Geometry: final body of the model. Coordinates: model frame, mm. Give positions to 0.01 mm unless a question says otherwise; leave off trailing zeros. Write each loop counter-clockwise with the first axis right and the second up, starting at its lowest first coordinate (ties: lowest second). Pieces come first, ordered by that corner, then holes. Notation, with made-up numbers: (78.25, 77.5) -> (125.25, 77.5) arc R13 cw to (125.25, 91.5) -> close; hole circle Ø5 at (-17.5, -35). An arc over 180 degrees is marked (long way). Answer in a Markdown table with one row per item. Add a question column.
Item 1: Section query B-B on x = 12.5. Output: boundary loops of the cut face in (y, z).
Item 2: Material intervals for probe 1 along Y at (x, z) = (18.25, -19.05); probe 2 along Z at (x, y) = (15, 402); probe 3 along Y at (x, z) = (1.5, -12), sorted ascending. Write a range as from..to.
Item 3: Section query A-A on y = 438.15. Output: boundary loops of the cut face in (x, z), plus the area to 3 significant figures.
Item 4: Section query C-C on z = -19.05. Output: boundary loops of the cut face in (x, y).
Item 5: First-contact query: P1, Ø10, axis at x = 8, z = -19.5, coming from the -Y side. Flat tip, straight axial feed; report the tip coordinate or a pass-through.
```python
from build123d import *

# Parameters (mm, degrees)
SKETCH1_W           = 19.05
SKETCH1_H           = 38.1
SKETCH1_W_2         = 15.875
SKETCH1_H_2         = 34.925
EXTRUDE_THIN1_DEPTH = 457.2
SKETCH3_W           = 19.05
SKETCH3_H           = 38.1
SKETCH3_W_2         = 15.875
SKETCH3_H_2         = 34.925
EXTRUDE_THIN2_DEPTH = 75.184
SKETCH4_R           = 14.2875
CUT_EXTRUDE1_DEPTH  = 20.05


with BuildPart() as part:
    # Sketch1 → Extrude-Thin1 (new body)
    with BuildSketch(Plane(origin=(0, 0, 0), x_dir=(1, 0, 0), z_dir=(0, 1, 0))):
        with Locations((9.525, 19.05)):
            Rectangle(SKETCH1_W, SKETCH1_H)
        with Locations((9.525, 19.05)):
            Rectangle(SKETCH1_W_2, SKETCH1_H_2, mode=Mode.SUBTRACT)
    extrude(amount=EXTRUDE_THIN1_DEPTH)

    # Sketch3 → Extrude-Thin2 (add)
    with BuildSketch(Plane(origin=(0, 0, 0), x_dir=(-1, 0, 0), z_dir=(0, -1, 0))):
        with Locations((-9.525, 19.05)):
            Rectangle(SKETCH3_W, SKETCH3_H)
        with Locations((-9.525, 19.05)):
            Rectangle(SKETCH3_W_2, SKETCH3_H_2, mode=Mode.SUBTRACT)
    extrude(amount=EXTRUDE_THIN2_DEPTH)

    # Sketch4 → Cut-Extrude1 (cut, through all)
    with BuildSketch(Plane(origin=(19.05, 0, 0), x_dir=(0, 0, -1), z_dir=(1, 0, 0))):
        with Locations((19.2024, 438.15)):
            Circle(SKETCH4_R)
        with Locations((19.05, 8.636)):
            Circle(SKETCH4_R)
    extrude(amount=-CUT_EXTRUDE1_DEPTH, mode=Mode.SUBTRACT)


solid = part.part
```
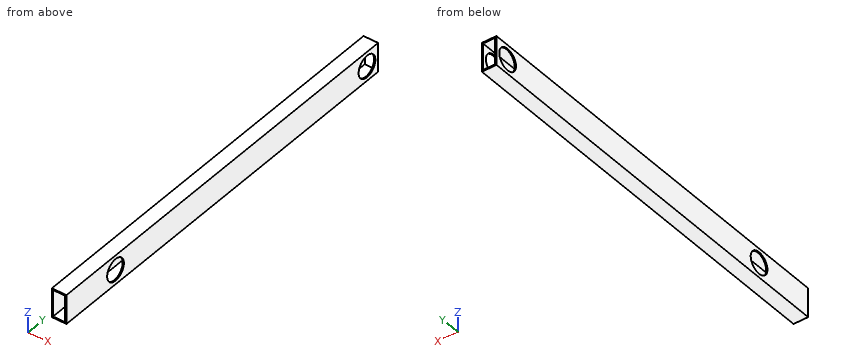
Findings below:
| question | item | result |
|---|---|---|
| 1 | outline | (-75.18, -38.1) -> (457.2, -38.1) -> (457.2, -36.51) -> (-75.18, -36.51) -> close; (-75.18, -1.59) -> (457.2, -1.59) -> (457.2, 0) -> (-75.18, 0) -> close |
| 2 | probe 1 | y = -75.18..-5.65, 22.92..423.86, 452.44..457.2 |
| 2 | probe 2 | z = -38.1..-36.51, -1.59..0 |
| 2 | probe 3 | y = -75.18..-3.79, 21.06..425.81, 450.49..457.2 |
| 3 | outline | (0, -38.1) -> (19.05, -38.1) -> (19.05, -33.49) -> (17.46, -33.49) -> (17.46, -36.51) -> (1.59, -36.51) -> (1.59, -33.49) -> (0, -33.49) -> close; (0, -4.91) -> (1.59, -4.91) -> (1.59, -1.59) -> (17.46, -1.59) -> (17.46, -4.91) -> (19.05, -4.91) -> (19.05, 0) -> (0, 0) -> close |
| 3 | area | 80.6 mm^2 |
| 4 | outline | (0, -75.18) -> (1.59, -75.18) -> (1.59, -5.65) -> (0, -5.65) -> close; (0, 22.92) -> (1.59, 22.92) -> (1.59, 423.86) -> (0, 423.86) -> close; (0, 452.44) -> (1.59, 452.44) -> (1.59, 457.2) -> (0, 457.2) -> close; (17.46, -75.18) -> (19.05, -75.18) -> (19.05, -5.65) -> (17.46, -5.65) -> close; (17.46, 22.92) -> (19.05, 22.92) -> (19.05, 423.86) -> (17.46, 423.86) -> close; (17.46, 452.44) -> (19.05, 452.44) -> (19.05, 457.2) -> (17.46, 457.2) -> close |
| 5 | P1 | passes through |
